from build123d import *

# Parameters (mm, degrees)
SZKIC1_W                    = 8
SZKIC1_H                    = 15
DODANIE_WYCI_GNI_CIE1_DEPTH = 10
ZAOKR_GLENIE1_R             = 4
SZKIC2_R                    = 1
DODANIE_WYCI_GNI_CIE2_DEPTH = 2
SZKIC4_R                    = 3
WYTNIJ_WYCI_GNI_CIE1_DEPTH  = 15
SZKIC9_R                    = 3
WYTNIJ_WYCI_GNI_CIE2_DEPTH  = 25


with BuildPart() as part:
    # Szkic1 → Dodanie-wyciągnięcie1 (new body)
    with BuildSketch(Plane.XY):
        Rectangle(SZKIC1_W, SZKIC1_H)
    extrude(amount=DODANIE_WYCI_GNI_CIE1_DEPTH)

    # Zaokrąglenie1
    zaokr_glenie1_edges = [part.edges().sort_by_distance(p)[0] for p in [
        (4, 7.5, 5),
        (-4, 7.5, 5),
    ]]
    fillet(zaokr_glenie1_edges, radius=ZAOKR_GLENIE1_R - 0.0001)  # a hair under: the kernel refuses the full size

    # Szkic2 → Dodanie-wyciągnięcie2 (add)
    with BuildSketch(Plane.XZ.offset(7.5)):
        with Locations(Location((-2, 5, 0), (0, 0, 90))):
            Circle(SZKIC2_R)
        with Locations(Location((2, 5, 0), (0, 0, 90))):
            Circle(SZKIC2_R)
    extrude(amount=DODANIE_WYCI_GNI_CIE2_DEPTH)

    # Szkic4 → Wytnij-wyciągnięcie1 (cut)
    with BuildSketch(Plane.XY.offset(10)):
        with Locations((0, 3.5)):
            Circle(SZKIC4_R)
    extrude(amount=-WYTNIJ_WYCI_GNI_CIE1_DEPTH, mode=Mode.SUBTRACT)

    # Szkic9 → Wytnij-wyciągnięcie2 (cut)
    with BuildSketch(Plane(origin=(0, -2.657422367, -5.349421519), x_dir=(1, 0, 0), z_dir=(0, -0.06975647374412577, 0.9975640502598243))):
        with Locations(Location((0, 0, 0), (0, 0, 90))):
            Circle(SZKIC9_R)
    extrude(amount=WYTNIJ_WYCI_GNI_CIE2_DEPTH, mode=Mode.SUBTRACT)


solid = part.part
Read the model definition and answer for the solid it produces. Units are mm, in the model's axes. A direction names the side the tool comes from. Coordinates: 2 decimals unless noted, no trailing zeros. Order: outer loops, then holes, each group sorted by start corner. A loop starts at its lowest first (then second) coordinate and runs counter-clockwise, first axis right, second up. Notation, with made-up numbers: (79, 38.5) - (113, 38.5) arc R24 ccw to (113, 53.5) - close; hole circle Ø6 at (-10.5, 68). An arc over 180 degrees is marked (long way). Use one line per item in the form item = value.
(1) Which of the six approach directions +Z, -Z, +X, -X, +Y, -Y give full straight-line access (tool end or side, diameter ignored) to faces 5 (the face through (2.6, -8.5, 4.2)), 6 (the face through (-1, 0, 0))?
Computed values:
face_5 = -Y
face_6 = -Z, +X, -X, +Y, -Y
(2) Straight lines are drawn through the part: L1, parallel to Y at x = -2.75, z = 3.5; L2, parallel to Y at x = -1.25, z = 6.75; L3, parallel to X at y = 6, z = 0.75. For each, find the intervals that lie inside material, in ascending order.
Computed values:
L1 = -7.5 to -4.48, -2.07 to 2.3, 4.7 to 6.4
L2 = -7.5 to -6.24, -0.77 to 0.77, 6.23 to 7.3
L3 = -3.12 to -1.66, 1.66 to 3.12
(3) Section B-B, the plane x = 2 is taken. Give the vertices of the cut face in (y, z).
Computed values:
outline = (-9.5, 4) - (-7.5, 4) - (-7.5, 0) - (-5.27, 0) - (-5.97, 10) - (-7.5, 10) - (-7.5, 6) - (-9.5, 6) - close; (-1.49, 10) - (-0.79, 0) - (1.26, 0) - (1.26, 10) - close; (5.74, 0) - (6.96, 0) - (6.96, 10) - (5.74, 10) - close
(4) Section C-C, the plane z = 1.25 is taken. Give the number of separate pieces and of enclosed holes in the cut face, then the cut area to 3 significant figures.
Computed values:
separate_pieces = 1
enclosed_holes = 2
area = 56.5 mm²
(5) Given pin 1 Ø1 at (x, y) = (-1, 1.5) entering from +Z, flat-ended and moving along its own axis, determine where the tip first touches the part or whether it passes through.
Computed values:
pin_1 = through
(6) For a pull along Y with two mould halves and no side action, classify faces 1 (the face through (2.859, 6.297, 5.07)), 2 (the face through (4, -2, 5)), 3 (the face through (-0.901, -0.522, 5.136)), 4 (the face through (-2, -9.5, 5)) as pulls with the +Y half, pulls with the -Y half, needs draft (parallel to the pull), parting line crosses it, or undercut.
Computed values:
face_1 = pulls with the +Y half
face_2 = needs draft
face_3 = undercut
face_4 = pulls with the -Y half
(7) Section A-A, the plane y = 5 is taken. Give the vertices of the cut face in (x, z).
Computed values:
outline = (-3.71, 0) - (-2.6, 0) - (-2.6, 10) - (-3.71, 10) - close; (2.6, 0) - (3.71, 0) - (3.71, 10) - (2.6, 10) - close
(8) Section D-D, the plane y = 3 is taken. Give the vertices of the cut face in (x, z).
Computed values:
outline = (-4, 0) - (-2.96, 0) - (-2.96, 10) - (-4, 10) - close; (2.96, 0) - (4, 0) - (4, 10) - (2.96, 10) - close
